from build123d import *

# Parameters (mm, degrees)
SKETCH_1_W          = 68
SKETCH_1_H          = 15
EXTRUDE_1_DEPTH     = 18
SKETCH_2_W          = 40
SKETCH_2_H          = 15
EXTRUDE_2_DEPTH     = 45
SKETCH_3_R          = 16
CUT_EXTRUDE_1_DEPTH = 43
SKETCH_4_R          = 16
SKETCH_4_R_2        = 14.3
EXTRUDE_3_DEPTH     = 2
SKETCH_5_R          = 2.75
CUT_EXTRUDE_2_DEPTH = 21


with BuildPart() as part:
    # 草图1 → 凸台-拉伸1 (new body)
    with BuildSketch(Plane.XY):
        Rectangle(SKETCH_1_W, SKETCH_1_H)
    extrude(amount=EXTRUDE_1_DEPTH)

    # 草图2 → 凸台-拉伸2 (add)
    with BuildSketch(Plane.XY.offset(18)):
        Rectangle(SKETCH_2_W, SKETCH_2_H)
    extrude(amount=EXTRUDE_2_DEPTH)

    # 草图3 → 切除-拉伸1 (cut)
    with BuildSketch(Plane.XZ.offset(7.5)):
        with Locations((0, 40)):
            Circle(SKETCH_3_R)
    extrude(amount=-CUT_EXTRUDE_1_DEPTH, mode=Mode.SUBTRACT)

    # 草图4 → 凸台-拉伸3 (add)
    with BuildSketch(Plane.XZ.offset(7.5)):
        with Locations(Location((0, 40, 0), (0, 0, 270))):
            Circle(SKETCH_4_R)
        with Locations(Location((0, 40, 0), (0, 0, 270))):
            Circle(SKETCH_4_R_2, mode=Mode.SUBTRACT)
    extrude(amount=-EXTRUDE_3_DEPTH)

    # 草图5 → 切除-拉伸2 (cut)
    with BuildSketch(Plane.XY.offset(18)):
        with Locations((28, 0)):
            Circle(SKETCH_5_R)
        with Locations((-28, 0)):
            Circle(SKETCH_5_R)
    extrude(amount=-CUT_EXTRUDE_2_DEPTH, mode=Mode.SUBTRACT)


solid = part.part
Input: part model. Units: mm. Frame: model coordinates. A direction names the side the tool comes from. Coordinates: 2 decimals unless noted, no trailing zeros. Order: outer loops, then holes, each group sorted by start corner. A loop starts at its lowest first (then second) coordinate and runs counter-clockwise, first axis right, second up. Notation, with made-up numbers: M -9,-29.5 L 21,-29.5 A14 cw 21,-11.5 Z; hole C 42,-5 d10. An arc over 180 degrees is marked long. Answer as CSV lines item,"result".
1. Section C-C (z = 40). Return the cut outline in (x, y), then the cut area to 3 significant figures.
Reported:
outline,"M -20,-7.5 L -14.3,-7.5 L -14.3,-5.5 L -16,-5.5 L -16,7.5 L -20,7.5 Z; M 14.3,-7.5 L 20,-7.5 L 20,7.5 L 16,7.5 L 16,-5.5 L 14.3,-5.5 Z"
area,"127 mm2"
2. Access query for faces 5 (the flat face through (0, 7.5, 17)), 6 (the cylindrical face through (25.253, 0.121, 9.126)), 7 (the flat face through (20, 0, 40)), 8 (the flat face through (-8.2, -5.5, 51.9)), 9 (the flat face through (-25.5, 1.8, 18)). Directions: +Z, -Z, +X, -X, +Y, -Y. A direction counts if a zero-diameter tool reaches every point of the face in a straight line with its end or side. Return the directions, or none.
Reported:
face 5,"+Z, -Z, +X, -X, +Y"
face 6,"+Z, -Z"
face 7,"+Z, +X, +Y, -Y"
face 8,"+Y"
face 9,"+Z, -X, +Y, -Y"
3. Section A-A (y = 0). Return the cut outline in (x, z).
Reported:
outline,"M -34,0 L -30.75,0 L -30.75,18 L -34,18 Z; M -25.25,0 L 25.25,0 L 25.25,18 L 20,18 L 20,63 L -20,63 L -20,18 L -25.25,18 Z; M 30.75,0 L 34,0 L 34,18 L 30.75,18 Z; hole C 0,40 d32"
4. Material intervals for line 1 (X direction, y = -6.85, z = 40); line 2 (Y direction, x = -28, z = 9); line 3 (X direction, y = 5.5, z = 20), sorted ascending. Write a range as from..to.
Reported:
line 1,"-20..-14.3, 14.3..20"
line 2,"-7.5..-2.75, 2.75..7.5"
line 3,"-20..20"
5. Pull-direction query (X, two-part tool) for faces 1 (the flat face through (34, 0, 9)), 2 (the flat face through (25, 2, 18)), 3 (the cylindrical face through (-30.747, 0.121, 9.126)), 4 (the flat face through (-34, 0, 9)); classes: released by +X, released by -X, zero draft, split by the parting line, or undercut.
Reported:
face 1,"released by +X"
face 2,"zero draft"
face 3,"undercut"
face 4,"released by -X"
6. Section D-D (y = 6). Return the cut outline in (x, z), then the cut area to 3 significant figures.
Reported:
outline,"M -34,0 L 34,0 L 34,18 L 20,18 L 20,63 L -20,63 L -20,18 L -34,18 Z; hole C 0,40 d32"
area,"2,220 mm2"
7. Section B-B (x = 28). Return the cut outline in (y, z).
Reported:
outline,"M -7.5,0 L -2.75,0 L -2.75,18 L -7.5,18 Z; M 2.75,0 L 7.5,0 L 7.5,18 L 2.75,18 Z"
8. First-contact query: P1, Ø8, axis at y = 5, z = 49, coming from the +X side; P2, Ø4.5, axis at y = 3.5, z = 39, coming from the -X side; P3, Ø4, axis at x = -30.5, y = -1.5, coming from the +Z side. Flat tips, straight axial feed; report the tip coordinate or a pass-through.
Reported:
P1,"x = 20"
P2,"x = -20"
P3,"z = 18"
